Source: CAD feature listing. Evaluate the final solid. Frame: model axes, mm. A direction names the side the tool comes from. Give positions to 0.01 mm unless a question says otherwise; leave off trailing zeros. Order: outer loops, then holes, each group sorted by start corner. A loop starts at its lowest first (then second) coordinate and runs counter-clockwise, first axis right, second up. Notation, with made-up numbers: M 55,63 L 105,63 A16 cw 105,89 Z; hole C 7,41 d9. An arc over 180 degrees is marked long. Return JSON: item names as keys, results as strings.
from build123d import *

# Parameters (mm, degrees)
F0_W           = 100
F0_H           = 50
F1_DEPTH       = 25
F2_R           = 10
F3_DEPTH       = 25
F5_D           = 8.8
F5_CBORE_D     = 14.25
F5_CBORE_DEPTH = 8


with BuildPart() as f1:
    # F0 (on Front) → F1 (new body)
    with BuildSketch(Plane.XZ):
        with Locations((50, -25)):
            Rectangle(F0_W, F0_H)
    extrude(amount=F1_DEPTH)

    # F2 (on face) → F3 (join)
    with BuildSketch(Plane.XZ.offset(25)):
        with Locations((80, -34)):
            Circle(F2_R)
    extrude(amount=F3_DEPTH)

    # F5 (through all)
    with Locations(Plane.XZ.offset(50)):
        with Locations((80, -34)):
            CounterBoreHole(F5_D / 2, F5_CBORE_D / 2, F5_CBORE_DEPTH)


solid = f1.part
1. Section query A-A (x = 80). Return loops of the section in (y, z) (3 decimals).
Evaluation:
{"outline": "M -50,-44 L -25,-44 L -25,-50 L 0,-50 L 0,-38.4 L -42,-38.4 L -42,-41.125 L -50,-41.125 Z; M -50,-26.875 L -42,-26.875 L -42,-29.6 L 0,-29.6 L 0,0 L -25,0 L -25,-24 L -50,-24 Z"}
2. Set-up query: faces 1 (the face through (49, -12, -50)), 2 (the face through (85, -42, -34)). Return all of +Z, -Z, +X, -X, +Y, -Y with unobstructed straight access to the full face (end or side cutting, diameter ignored); none if empty.
Evaluation:
{"face 1": "-Z, +X, -X, +Y, -Y", "face 2": "-Y"}
3. Section query C-C (y = -43.5). Return loops of the section in (x, z) (3 decimals), then the cut area to 3 significant figures.
Evaluation:
{"outline": "C 80,-34 d20; hole C 80,-34 d14.25", "area": "155 mm^2"}
4. Draft query along Z for faces 3 (the face through (72, -37, -40)), 4 (the face through (86.58, -46.06, -36.73)), 5 (the face through (49, -25, -25)). Return one class per face: pulls with the +Z half, pulls with the -Z half, needs draft (parallel to the pull), parting line crosses it, or undercut.
Evaluation:
{"face 3": "parting line crosses it", "face 4": "undercut", "face 5": "needs draft"}
5. Section query B-B (z = -34). Return loops of the section in (x, y) (3 decimals).
Evaluation:
{"outline": "M 0,-25 L 70,-25 L 70,-50 L 72.875,-50 L 72.875,-42 L 75.6,-42 L 75.6,0 L 0,0 Z; M 84.4,-42 L 87.125,-42 L 87.125,-50 L 90,-50 L 90,-25 L 100,-25 L 100,0 L 84.4,0 Z"}
6. First-contact query: pin 1 (4 mm diameter, centred on y = -35.5, z = -44, fed in from +X); pin 2 (7 mm diameter, centred on x = 81.5, z = -31, fed in from -Y); pin 3 (1 mm diameter, centred on x = 34, z = -14.5, fed in from -Y). Flat tips, straight axial feed; report the tip coordinate or a pass-through.
Evaluation:
{"pin 1": "stops at x = 86", "pin 2": "stops at y = -42", "pin 3": "stops at y = -25"}
7. Section query D-D (z = -4). Return loops of the section in (x, y).
Evaluation:
{"outline": "M 0,-25 L 100,-25 L 100,0 L 0,0 Z"}
8. Ray query, probe 1 along Z at (x, y) = (80, -45.5) (3 decimals); probe 2 along Y at (x, z) = (22.5, -36.5); probe 3 along Y at (x, z) = (74.5, -34). Return the intervals inside material, ascending.
Evaluation:
{"probe 1": "z = -44 to -41.125, -26.875 to -24", "probe 2": "y = -25 to 0", "probe 3": "y = -42 to 0"}
